Model file for the job. Use its own axes, mm. Face numbers are marked on the shaded views. A direction names the side the tool comes from. Coordinates: 2 decimals unless noted, no trailing zeros. Write each loop counter-clockwise with the first axis right and the second up, starting at its lowest first coordinate (ties: lowest second). Pieces come first, ordered by that corner, then holes. Notation, with made-up numbers: M 18,62.5 L 29,62.5 A20 ccw 29,79.5 Z; hole C 22,-17 d10. An arc over 180 degrees is marked long. One line per question, with ' | ' between items. Start each with the question number.
(1) Tool access for the marked faces 1, 2 and 3: list every direction of +Z, -Z, +X, -X, +Y, -Y with a clear straight run to the whole face (end or side of a thin tool).
(2) Flat gauge pins, fed straight in: pin 1 Ø3 at (x, z) = (-1, 3) entering from +Y; pin 2 Ø4 at (y, z) = (1, -30.5) entering from -X; pin 3 Ø4.5 at (x, z) = (1, 3) entering from -Y; pin 4 Ø1 at (y, z) = (3.5, -41.5) entering from -X. Where does each tip first touch, or does it go through?
(3) Cut at C-C (z = -10.5). Write the cut outline in (x, y).
(4) Wall check: probe 1 along X at (y, z) = (0, -27); probe 2 along Z at (x, y) = (1, -0.5). Give the ranges that are in metal, low to high.
from build123d import *

# Parameters (mm, degrees)
ESQUISSE1_R        = 4
BOSS_EXTRU_1_DEPTH = 6
ESQUISSE2_R        = 5
BOSS_EXTRU_2_DEPTH = 4
CONG_1_R           = 1
ESQUISSE3_W        = 5
ESQUISSE3_H        = 5
BOSS_EXTRU_3_DEPTH = 60
BOSS_EXTRU_4_START = 2.5
ESQUISSE4_R        = 4
BOSS_EXTRU_4_DEPTH = 2.5


with BuildPart() as part:
    # Esquisse1 → Boss.-Extru.1 (new body)
    with BuildSketch(Plane.XY):
        Circle(ESQUISSE1_R)
        with BuildLine():
            Line((-2, 1.5), (2, 1.5))
            ThreePointArc((2, 1.5), (2.5, 0), (2, -1.5))
            Line((2, -1.5), (-2, -1.5))
            ThreePointArc((-2, -1.5), (-2.5, 0), (-2, 1.5))
        make_face(mode=Mode.SUBTRACT)
    extrude(amount=BOSS_EXTRU_1_DEPTH)

    # Esquisse2 → Boss.-Extru.2 (add)
    with BuildSketch(Plane(origin=(0, 0, 0), x_dir=(-1, 0, 0), z_dir=(0, 0, -1))):
        Circle(ESQUISSE2_R)
    extrude(amount=BOSS_EXTRU_2_DEPTH)

    # Congé1
    cong_1_edges = [part.edges().sort_by_distance(p)[0] for p in [
        (5, 0, 0),
    ]]
    fillet(cong_1_edges, radius=CONG_1_R - 0.0001)  # a hair under: the kernel refuses the full size

    # Esquisse3 → Boss.-Extru.3 (add)
    with BuildSketch(Plane(origin=(0, 0, -4), x_dir=(-1, 0, 0), z_dir=(0, 0, -1))):
        Rectangle(ESQUISSE3_W, ESQUISSE3_H)
    extrude(amount=BOSS_EXTRU_3_DEPTH)

    # Esquisse4 → Boss.-Extru.4 (add)
    with BuildSketch(Plane(origin=(0, 0, -4), x_dir=(-1, 0, 0), z_dir=(0, 0, -1)).offset(BOSS_EXTRU_4_START)):
        with Locations(Location((0, 0, 0), (0, 0, 180))):
            Circle(ESQUISSE4_R)
    extrude(amount=-BOSS_EXTRU_4_DEPTH)


solid = part.part
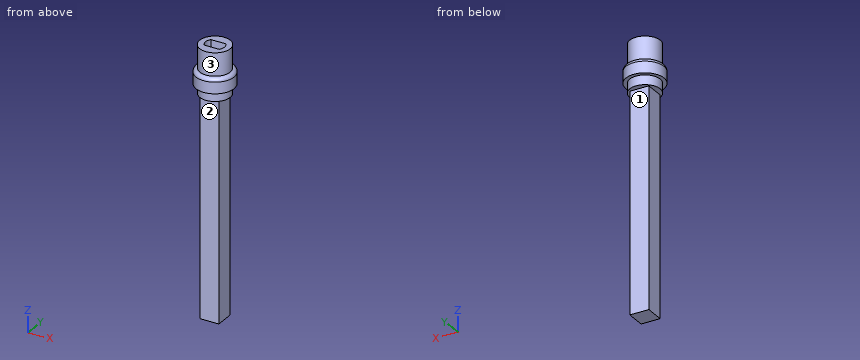
Filled in:
1) face 1: -Z, +X, -X, +Y | face 2: -Z, +X, -X, -Y | face 3: +Z
2) pin 1: y = 4 | pin 2: x = -2.5 | pin 3: y = -4 | pin 4: through
3) outline: M -2.5,-2.5 L 2.5,-2.5 L 2.5,2.5 L -2.5,2.5 Z
4) probe 1: -2.5 to 2.5 | probe 2: -64 to 0
